Model file for the job. Use its own axes, mm. Face numbers are marked on the shaded views. A direction names the side the tool comes from. Coordinates: 2 decimals unless noted, no trailing zeros. Loops run counter-clockwise (first coordinate to the right, second up) from the corner with the lowest first, then second, coordinate; pieces in that order, holes last.
from build123d import *

# Parameters (mm, degrees)
SKETCH2_W               = 150
SKETCH2_H               = 75
BOSS_EXTRUDE1_DEPTH     = 12.5
SKETCH3_W               = 75
SKETCH3_H               = 50
BOSS_EXTRUDE3_DEPTH     = 25
SKETCH4_W               = 50
SKETCH4_H               = 24
CUT_EXTRUDE1_DEPTH      = 25
CUT_EXTRUDE1_DRAFT      = -5
SKETCH5_W               = 18
SKETCH5_H               = 10
CUT_EXTRUDE2_DEPTH      = 88.5
MIRROR2_COPY_1_SKETCH_W = 18
MIRROR2_COPY_1_SKETCH_H = 10
MIRROR2_COPY_1_DEPTH    = 88.5
RIB1_REACH              = 93.856
SKETCH6_WALL_W          = 230.781121652
SKETCH6_WALL_H          = 10


with BuildPart() as part:
    # Sketch2 → Boss-Extrude1 (new, symmetric)
    with BuildSketch(Plane(origin=(0, 0, 0), x_dir=(1, 0, 0), z_dir=(0, 1, 0))):
        Rectangle(SKETCH2_W, SKETCH2_H)
    extrude(amount=BOSS_EXTRUDE1_DEPTH, both=True)

    # Sketch3 → Boss-Extrude3 (add)
    with BuildSketch(Plane(origin=(0, 12.5, 0), x_dir=(1, 0, 0), z_dir=(0, 1, 0))):
        Rectangle(SKETCH3_W, SKETCH3_H)
    extrude(amount=BOSS_EXTRUDE3_DEPTH)


with BuildPart() as cut_extrude1_tool:
    # Sketch4 → Cut-Extrude1 (with draft: the straight prism first)
    with BuildSketch(Plane(origin=(0, 37.5, 0), x_dir=(1, 0, 0), z_dir=(0, 1, 0))):
        Rectangle(SKETCH4_W, SKETCH4_H)
    extrude(amount=-CUT_EXTRUDE1_DEPTH)
    # Cut-Extrude1: the draft: its side faces are tilted about the plane it starts from
    cut_extrude1_sides = [cut_extrude1_tool.faces().sort_by_distance(p)[0] for p in [
        (-25, 25, 0),
        (0, 25, 12),
        (25, 25, 0),
        (0, 25, -12),
    ]]
    draft(cut_extrude1_sides, Plane(origin=(0, 37.5, 0), x_dir=(1, 0, 0), z_dir=(0, 1, 0)), CUT_EXTRUDE1_DRAFT)


with BuildPart() as part_1:
    add(part.part)

    # Cut-Extrude1: cut by cut_extrude1_tool
    add(cut_extrude1_tool.part, mode=Mode.SUBTRACT)

    # Sketch5 → Cut-Extrude2 (cut, through all)
    with BuildSketch(Plane(origin=(0, 12.5, 0), x_dir=(1, 0, 0), z_dir=(0, 1, 0))):
        with Locations((55, -21.5)):
            Rectangle(SKETCH5_W, SKETCH5_H)
    cut_extrude2 = extrude(amount=-CUT_EXTRUDE2_DEPTH, mode=Mode.SUBTRACT)

    # Mirror1: Cut-Extrude2 across plane
    add(cut_extrude2.mirror(Plane(origin=(0, 0, 0), x_dir=(0, 0, 1), z_dir=(1, 0, 0))), mode=Mode.SUBTRACT)

    # Mirror2: Cut-Extrude2 across plane
    add(cut_extrude2.mirror(Plane.XY), mode=Mode.SUBTRACT)

    # Mirror2 copy 1 sketch → Mirror2 copy 1 (cut, through all)
    with BuildSketch(Plane(origin=(0, 12.5, 0), x_dir=(-1, 0, 0), z_dir=(0, 1, 0))):
        with Locations((55, -21.5)):
            Rectangle(MIRROR2_COPY_1_SKETCH_W, MIRROR2_COPY_1_SKETCH_H)
    extrude(amount=-MIRROR2_COPY_1_DEPTH, mode=Mode.SUBTRACT)

    # Sketch6 wall → Rib1 (add, up to next)
    with BuildSketch(Plane(origin=(-56.25, 25, 0), x_dir=(0.832050294338, 0.554700196225, 0), z_dir=(-0.554700196225, 0.832050294338, 0)), mode=Mode.PRIVATE) as rib1_sk1:
        Rectangle(SKETCH6_WALL_W, SKETCH6_WALL_H)
    rib1_tool1 = extrude(rib1_sk1.sketch, amount=-RIB1_REACH, mode=Mode.PRIVATE) - part_1.part
    rib1 = rib1_tool1.solids().sort_by_distance((-56.25, 25, 0))[0]
    add(rib1)

    # Mirror3: Rib1 across plane
    add(rib1.mirror(Plane(origin=(0, 0, 0), x_dir=(0, 0, 1), z_dir=(1, 0, 0))))


solid = part_1.part
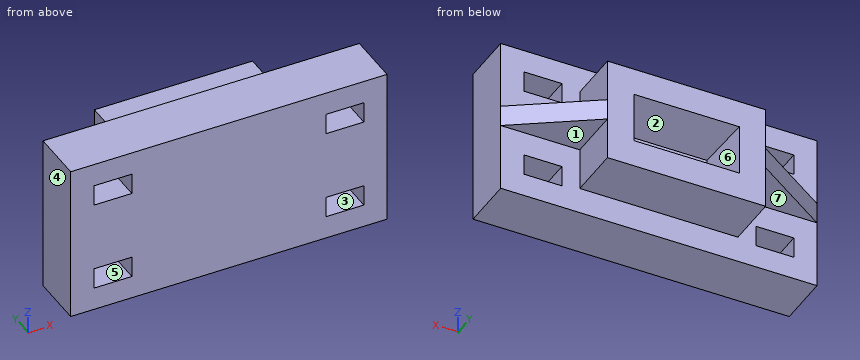
Q1. Mould opens along X. For the marked faces 4, 5, 6 and 7 say: +X half, -X half, draft (parallel to the pull), parting line (faces both ways), or undercut.
Answers:
face 4: -X half
face 5: undercut
face 6: undercut
face 7: draft
Q2. Flat gauge pins, fed straight in: P1, Ø7.5, axis at x = 56.5, y = 26, coming from the -Z side; P2, Ø12.5, axis at x = -13, y = 25, coming from the +Z side; P3, Ø5, axis at x = 45, z = -4, coming from the +Y side. Where does each tip first touch, or does it go through?
Answers:
P1: stops at z = -5
P2: stops at z = 25
P3: stops at y = 34.17
Q3. Slice it at B-B (y = -1.5). List the corners of the cut face in (x, z).
Answers:
outline: (-75, -37.5) - (75, -37.5) - (75, 37.5) - (-75, 37.5) - close; hole (-64, -26.5) - (-46, -26.5) - (-46, -16.5) - (-64, -16.5) - close; hole (-64, 16.5) - (-46, 16.5) - (-46, 26.5) - (-64, 26.5) - close; hole (46, -26.5) - (64, -26.5) - (64, -16.5) - (46, -16.5) - close; hole (46, 16.5) - (64, 16.5) - (64, 26.5) - (46, 26.5) - close
Q4. Which spindle directions (+Z, -Z, +X, -X, +Y, -Y) get a long thin tool onto all of the face, cutting with end or side? Do the marked faces 1, 2 and 3. Say none if no direction does.
Answers:
face 1: -Z, +X, +Y
face 2: +Y
face 3: +Y, -Y
Q5. Drill centre lines: line 1 (X direction, y = 6, z = -18.5); line 2 (Z direction, x = -55, y = 25); line 3 (X direction, y = 15, z = -14). Where is each one in solid material? Low to high.
Answers:
line 1: x = -75 to -64, -46 to 46, 64 to 75
line 2: z = -5 to 5
line 3: x = -37.5 to 37.5
Q6. Slice it at D-D (x = -19). List the corners of the cut face in (y, z).
Answers:
outline: (-12.5, -37.5) - (12.5, -37.5) - (12.5, -25) - (37.5, -25) - (37.5, -12) - (12.5, -9.81) - (12.5, 9.81) - (37.5, 12) - (37.5, 25) - (12.5, 25) - (12.5, 37.5) - (-12.5, 37.5) - close
Q7. Slice it at C-C (x = -50). List the corners of the cut face in (y, z), and give its area (3 significant figures).
Answers:
outline: (-12.5, -37.5) - (12.5, -37.5) - (12.5, -26.5) - (-12.5, -26.5) - close; (-12.5, -16.5) - (12.5, -16.5) - (12.5, -5) - (29.17, -5) - (29.17, 5) - (12.5, 5) - (12.5, 16.5) - (-12.5, 16.5) - close; (-12.5, 26.5) - (12.5, 26.5) - (12.5, 37.5) - (-12.5, 37.5) - close
area: 1,540 mm2
Q8. Slice it at A-A (z = 22). List the corners of the cut face in (x, y), and give its area (4 significant figures).
Answers:
outline: (-75, -12.5) - (-64, -12.5) - (-64, 12.5) - (-75, 12.5) - close; (-46, -12.5) - (46, -12.5) - (46, 12.5) - (37.5, 12.5) - (37.5, 37.5) - (-37.5, 37.5) - (-37.5, 12.5) - (-46, 12.5) - close; (64, -12.5) - (75, -12.5) - (75, 12.5) - (64, 12.5) - close
area: 4,725 mm2
